Autodesk Inventor part; units mm, degrees
ref_plane "YZ Plane" through (0, 0, 0) normal (1, 0, 0) x (0, 1, 0)
ref_plane "XZ Plane" through (0, 0, 0) normal (0, 1, 0) x (-1, 0, 0)
ref_plane "XY Plane" through (0, 0, 0) normal (0, 0, 1) x (1, 0, 0)
sketch "Sketch1" plane through (0, 0, 0) normal (0, 1, 0) x (-1, 0, 0)
  circle A0 centre (0, 0) radius 22.5
  dimension "d0" = 45
extrude "Extrusion1" add sketch "Sketch1" along normal blind 5
sketch "Sketch2" plane through (0, 5, 0) normal (0, 1, 0) x (1, 0, 0)
  circle A0 centre (0, 0) radius 19.75
  circle A1 centre (0, 0) radius 18.5
  dimension "d3" = 39.5
  dimension "d4" = 37
extrude "Extrusion2" add sketch "Sketch2" along normal blind 5
sketch "Sketch3" plane through (0, 0, 0) normal (0, -1, 0) x (1, 0, 0)
  circle A0 centre (0, 0) radius 14.5
  dimension "d7" = 29
extrude "Extrusion3" cut sketch "Sketch3" against normal blind 3
sketch "Sketch4" plane through (0, 3, 0) normal (0, -1, 0) x (1, 0, 0)
  circle A0 centre (0, 0) radius 11
  dimension "d10" = 22
extrude "Extrusion4" cut sketch "Sketch4" against normal blind 5
properties part number "Button_Holder"
Part model, mm, in its own coordinate system. A direction names the side the tool comes from. Round coordinates to 2 decimals unless told otherwise and drop trailing zeros. Write each loop counter-clockwise with the first axis right and the second up, starting at its lowest first coordinate (ties: lowest second). Pieces come first, ordered by that corner, then holes. Notation, with made-up numbers: (-24.75, 71) - (7.25, 71) arc R19 ccw to (7.25, 84) - close; hole circle Ø1 at (53.5, 2). An arc over 180 degrees is marked (long way). Use CSV: the item, a comma, the result in double quotes.
Item 1: Slice it at B-B, the plane z = -10. Write the cut outline in (x, y), then the cut area to 3 significant figures.
Results list:
outline,"(-20.16, 0) - (-10.5, 0) - (-10.5, 3) - (-4.58, 3) - (-4.58, 5) - (-15.56, 5) - (-15.56, 10) - (-17.03, 10) - (-17.03, 5) - (-20.16, 5) - close; (4.58, 3) - (10.5, 3) - (10.5, 0) - (20.16, 0) - (20.16, 5) - (17.03, 5) - (17.03, 10) - (15.56, 10) - (15.56, 5) - (4.58, 5) - close"
area,"135 mm²"
Item 2: Slice it at C-C, the plane y = 6. Write the cut outline in (x, z), then the cut area to 3 significant figures.
Results list:
outline,"circle Ø39.5 at (0, 0); hole circle Ø37 at (0, 0)"
area,"150 mm²"
Item 3: Flat gauge pins, fed straight in: P1, Ø6, axis at x = 1, y = 4.5, coming from the +Z side; P2, Ø11, axis at x = -0.5, z = 2, coming from the +Y side; P3, Ø22.5, axis at x = 2, z = -1, coming from the +Y side. Where does each tip first touch, or does it go through?
Results list:
P1,"stops at z = 22.5"
P2,"passes through"
P3,"stops at y = 5"
Item 4: Tool access for faces 1 (the flat face through (-18, 10, 6)), 2 (the cylindrical face through (-4.01, 7.46, -18.06)), 3 (the cylindrical face through (6.691, 1.479, -12.864)): list every direction of +Z, -Z, +X, -X, +Y, -Y with a clear straight run to the whole face (end or side of a thin tool).
Results list:
face 1,"+Z, -Z, +X, -X, +Y"
face 2,"+Y"
face 3,"-Y"
Item 5: Slice it at A-A, the plane x = 0. Write the cut outline in (y, z).
Results list:
outline,"(0, -22.5) - (5, -22.5) - (5, -19.75) - (10, -19.75) - (10, -18.5) - (5, -18.5) - (5, -11) - (3, -11) - (3, -14.5) - (0, -14.5) - close; (0, 14.5) - (3, 14.5) - (3, 11) - (5, 11) - (5, 18.5) - (10, 18.5) - (10, 19.75) - (5, 19.75) - (5, 22.5) - (0, 22.5) - close"
Item 6: Pull direction Z, two halves, no side cores. Call faces 4 (the cylindrical face through (-10.382, 2.465, 19.961)), 5 (the flat face through (0, 0, -15)), 6 (the flat face through (-8, 5, -8)): pulls with the +Z half, pulls with the -Z half, needs draft (parallel to the pull), parting line crosses it, or undercut.
Results list:
face 4,"parting line crosses it"
face 5,"needs draft"
face 6,"undercut"
Item 7: Wall check: L1, parallel to X at y = 4.75, z = 0.5; L2, parallel to Z at x = 0, y = 0.8; L3, parallel to X at y = 6.9, z = 0. Give the ranges that are in metal, low to high.
Results list:
L1,"x = -22.49 to -10.99, 10.99 to 22.49"
L2,"z = -22.5 to -14.5, 14.5 to 22.5"
L3,"x = -19.75 to -18.5, 18.5 to 19.75"
Item 8: Slice it at D-D, the plane z = -15.5. Write the cut outline in (x, y), then the cut area to 3 significant figures.
Results list:
outline,"(-16.31, 0) - (16.31, 0) - (16.31, 5) - (12.24, 5) - (12.24, 10) - (10.1, 10) - (10.1, 5) - (-10.1, 5) - (-10.1, 10) - (-12.24, 10) - (-12.24, 5) - (-16.31, 5) - close"
area,"184 mm²"
